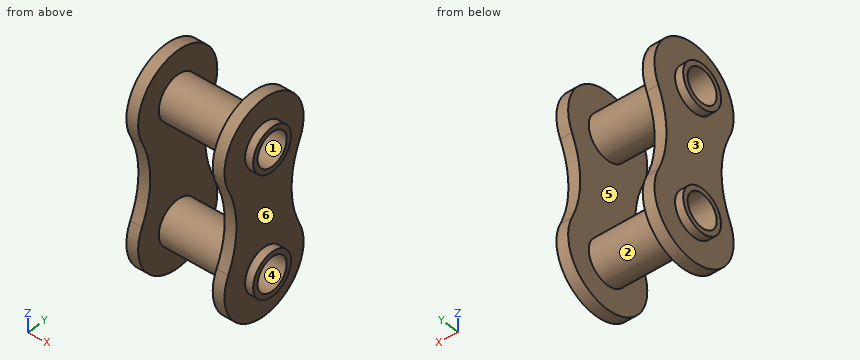
from build123d import *

# Parameters (mm, degrees)
SKETCH_1_R        = 6.8
SKETCH_1_R_2      = 5.22
EXTRUDE_1_DEPTH   = 18
EXTRUDE_1_2_DEPTH = 18
EXTRUDE_START     = 15.45
SKETCH_3_R        = 6.8
EXTRUDE_3_DEPTH   = 3.7


with BuildPart() as part:
    # Sketch 1 → Extrude 1 (new, symmetric)
    with BuildSketch(Plane(origin=(0, 0, 0), x_dir=(0, 0, -1), z_dir=(1, 0, 0))):
        with Locations((-19.05, 0)):
            Circle(SKETCH_1_R)
        with Locations((-19.05, 0)):
            Circle(SKETCH_1_R_2, mode=Mode.SUBTRACT)
    extrude(amount=EXTRUDE_1_DEPTH, both=True)



with BuildPart() as body_2:
    # Sketch 1 → Extrude 1 2 (new, symmetric)
    with BuildSketch(Plane(origin=(0, 0, 0), x_dir=(0, 0, -1), z_dir=(1, 0, 0))):
        with Locations((19.05, 0)):
            Circle(SKETCH_1_R)
        with Locations((19.05, 0)):
            Circle(SKETCH_1_R_2, mode=Mode.SUBTRACT)
    extrude(amount=EXTRUDE_1_2_DEPTH, both=True)


with BuildPart() as part_1:
    add(part.part)

    add(body_2.part)  # Extrude 3 merges body 2
    # Sketch 3 → Extrude 3 (add)
    with BuildSketch(Plane(origin=(0, 0, 0), x_dir=(0, 0, -1), z_dir=(1, 0, 0)).offset(EXTRUDE_START)):
        with BuildLine():
            ThreePointArc((-12.929864253, 12.813428052), (-33.25, 0), (-12.929864253, -12.813428052))
            ThreePointArc((-12.929864253, -12.813428052), (0, -9.884050697), (12.929864253, -12.813428052))
            ThreePointArc((12.929864253, -12.813428052), (33.25, 0), (12.929864253, 12.813428052))
            ThreePointArc((12.929864253, 12.813428052), (0, 9.884050697), (-12.929864253, 12.813428052))
        make_face()
        with Locations((-19.05, 0)):
            Circle(SKETCH_3_R, mode=Mode.SUBTRACT)
        with Locations((19.05, 0)):
            Circle(SKETCH_3_R, mode=Mode.SUBTRACT)
    extrude_3 = extrude(amount=-EXTRUDE_3_DEPTH)

    # Mirror 1: Extrude 3 across plane
    add(extrude_3.mirror(Plane(origin=(0, 0, 0), x_dir=(0, 0, 1), z_dir=(1, 0, 0))))


solid = part_1.part
Check sheet for the modelled part. Datum: model origin and axes. Units: mm. Face numbers are marked on the shaded views. A direction names the side the tool comes from. Coordinates: 2 decimals unless noted, no trailing zeros. Write each loop counter-clockwise with the first axis right and the second up, starting at its lowest first coordinate (ties: lowest second). Pieces come first, ordered by that corner, then holes. Notation, with made-up numbers: M 8.5,39.5 L 34.5,39.5 A20 ccw 34.5,67.5 Z; hole C 60,12 d11. An arc over 180 degrees is marked long. Answer as CSV lines item,"result".
Q1. Set-up check for the marked faces 1 and 2: record each of +Z, -Z, +X, -X, +Y, -Y from which the full face is reachable in a straight line by a thin tool's end or side.
Check result:
face 1,"+X, -X"
face 2,"none"
Q2. Cross-section at B-B (x = 9.5). Record the boundary of the cut face in (y, z), then the cut area to 3 significant figures.
Check result:
outline,"C 0,-19.05 d13.6; C 0,19.05 d13.6; hole C 0,-19.05 d10.44; hole C 0,19.05 d10.44"
area,"119 mm^2"
Q3. Go/stop test with flat-tipped pins: pin 1 (5 mm diameter, centred on x = -10, y = -1.5, fed in from +Z); pin 2 (4 mm diameter, centred on x = -8.5, z = -24.5, fed in from +Y); pin 3 (12 mm diameter, centred on y = -7.5, z = 2.5, fed in from +X); pin 4 (3 mm diameter, centred on x = 9.5, y = 6, fed in from +Z). Record where each tip stops, or that it passes through.
Check result:
pin 1,"z = 33.25"
pin 2,"y = 5.86"
pin 3,"x = 15.45"
pin 4,"z = 24.15"
Q4. Mould release check, pull along X, two halves, no side actions. Record for the marked faces 3, 4, 5 and 6: released by +X, released by -X, zero draft, split by the parting line, or undercut.
Check result:
face 3,"released by -X"
face 4,"zero draft"
face 5,"undercut"
face 6,"released by +X"
Q5. Material ranges on probe 1 along X at (y, z) = (-7, 16.5); probe 2 along Y at (x, z) = (3.5, -19.05); probe 3 along Z at (x, y) = (-10.5, 4.75), recorded low to high. Write a range as from..to.
Check result:
probe 1,"-15.45..-11.75, 11.75..15.45"
probe 2,"-6.8..-5.22, 5.22..6.8"
probe 3,"-23.92..-21.21, -16.89..-14.18, 14.18..16.89, 21.21..23.92"
Q6. Cross-section at C-C (y = 0). Count the separate pieces of the cut face and the enclosed holes in it, then the cut area to 3 significant figures.
Check result:
separate pieces,"3"
enclosed holes,"1"
area,"518 mm^2"
Q7. Cross-section at D-D (y = 11.5). Record the boundary of the cut face in (x, z), then the cut area to 3 significant figures.
Check result:
outline,"M -15.45,-27.38 L -11.75,-27.38 L -11.75,-9.71 L -15.45,-9.71 Z; M -15.45,9.71 L -11.75,9.71 L -11.75,27.38 L -15.45,27.38 Z; M 11.75,-27.38 L 15.45,-27.38 L 15.45,-9.71 L 11.75,-9.71 Z; M 11.75,9.71 L 15.45,9.71 L 15.45,27.38 L 11.75,27.38 Z"
area,"261 mm^2"
Q8. Cross-section at A-A (z = 19.05). Record the boundary of the cut face in (x, y).
Check result:
outline,"M -18,-6.8 L -15.45,-6.8 L -15.45,-14.2 L -11.75,-14.2 L -11.75,-6.8 L 11.75,-6.8 L 11.75,-14.2 L 15.45,-14.2 L 15.45,-6.8 L 18,-6.8 L 18,-5.22 L -18,-5.22 Z; M -18,5.22 L 18,5.22 L 18,6.8 L 15.45,6.8 L 15.45,14.2 L 11.75,14.2 L 11.75,6.8 L -11.75,6.8 L -11.75,14.2 L -15.45,14.2 L -15.45,6.8 L -18,6.8 Z"
